from build123d import *

# Parameters (mm, degrees)
SKETCH1_W           = 22
SKETCH1_H           = 37
SKETCH1_R           = 2.5
SKETCH1_W_2         = 12
SKETCH1_H_2         = 10
BOSS_EXTRUDE2_DEPTH = 6
CUT_EXTRUDE2_DEPTH  = 6


with BuildPart() as part:
    # Sketch1 → Boss-Extrude2 (new body)
    with BuildSketch(Plane.XY):
        Rectangle(SKETCH1_W, SKETCH1_H)
        with Locations((-7, 14.5)):
            Circle(SKETCH1_R, mode=Mode.SUBTRACT)
        with Locations((7, 14.5)):
            Circle(SKETCH1_R, mode=Mode.SUBTRACT)
        with Locations((0, -12)):
            Rectangle(SKETCH1_W_2, SKETCH1_H_2, mode=Mode.SUBTRACT)
    extrude(amount=BOSS_EXTRUDE2_DEPTH)

    # Sketch3 → Cut-Extrude2 (cut)
    with BuildSketch(Plane(origin=(0, 0, 0), x_dir=(-1, 0, 0), z_dir=(0, 0, -1))):
        Polygon((0, -17), (-3, -17), (-3, -18.5), (0, -18.5), (3, -18.5), (3, -17), align=None)
    extrude(amount=-CUT_EXTRUDE2_DEPTH, mode=Mode.SUBTRACT)


solid = part.part
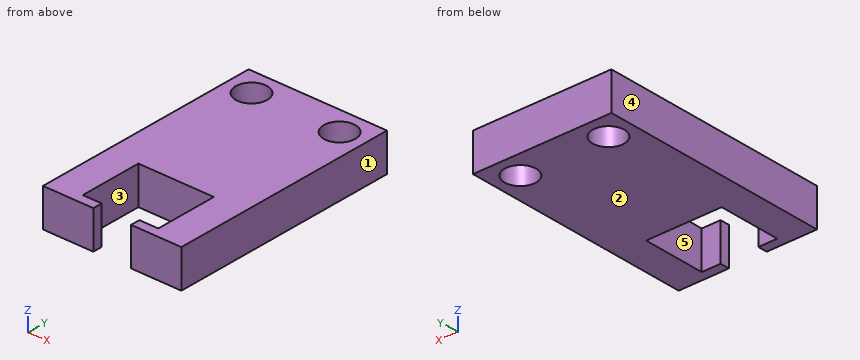
The listing builds one solid part. Answer for the finished solid, in the listing's coordinates (mm). Face numbers are marked on the shaded views. A direction names the side the tool comes from. Give positions to 0.01 mm unless a question says otherwise; leave off trailing zeros. Write each loop counter-clockwise with the first axis right and the second up, starting at its lowest first coordinate (ties: lowest second). Pieces come first, ordered by that corner, then holes. Notation, with made-up numbers: (-36, 8.5) -> (19, 8.5) arc R10 cw to (19, 23.5) -> close; hole circle Ø3 at (32, 43.25). An arc over 180 degrees is marked (long way). One line per question, with ' | ' between items. Start each with the question number.
1. Given pin 1 Ø6 at (x, y) = (-7, 14.5) entering from +Z, flat-ended and moving along its own axis, determine where the tip first touches the part or whether it passes through.
2. Section C-C (z = 1.6) is taken. Determine the outline of the cut face in (x, y), plus the area to 3 significant figures.
3. Section D-D (y = 14.5) is taken. Determine the outline of the cut face in (x, z), plus the area to 3 significant figures.
4. Find the intervals of material crossed by probe 1 along Y at (x, z) = (7, 1.2); probe 2 along X at (y, z) = (15.5, 1.7); probe 3 along X at (y, z) = (14, 4.2), in increasing order.
5. For a pull along X with two mould halves and no side action, classify the marked faces 1, 2 and 3 as pulls with the +X half, pulls with the -X half, needs draft (parallel to the pull), parting line crosses it, or undercut.
6. Section B-B (x = 7) is taken. Determine the outline of the cut face in (y, z), plus the area to 3 significant figures.
7. Section A-A (y = -10) is taken. Determine the outline of the cut face in (x, z).
8. For the marked faces 4 and 5, determine the directions among +Z, -Z, +X, -X, +Y, -Y from which every point of the face is accessible in a straight line to the end or side of a thin tool.
Response values:
1) pin 1: z = 6
2) outline: (-11, -18.5) -> (-3, -18.5) -> (-3, -17) -> (-6, -17) -> (-6, -7) -> (6, -7) -> (6, -17) -> (3, -17) -> (3, -18.5) -> (11, -18.5) -> (11, 18.5) -> (-11, 18.5) -> close; hole circle Ø5 at (-7, 14.5); hole circle Ø5 at (7, 14.5) | area: 646 mm2
3) outline: (-11, 0) -> (-9.5, 0) -> (-9.5, 6) -> (-11, 6) -> close; (-4.5, 0) -> (4.5, 0) -> (4.5, 6) -> (-4.5, 6) -> close; (9.5, 0) -> (11, 0) -> (11, 6) -> (9.5, 6) -> close | area: 72.0 mm2
4) probe 1: -18.5 to 12, 17 to 18.5 | probe 2: -11 to -9.29, -4.71 to 4.71, 9.29 to 11 | probe 3: -11 to -9.45, -4.55 to 4.55, 9.45 to 11
5) face 1: pulls with the +X half | face 2: needs draft | face 3: undercut
6) outline: (-18.5, 0) -> (12, 0) -> (12, 6) -> (-18.5, 6) -> close; (17, 0) -> (18.5, 0) -> (18.5, 6) -> (17, 6) -> close | area: 192 mm2
7) outline: (-11, 0) -> (-6, 0) -> (-6, 6) -> (-11, 6) -> close; (6, 0) -> (11, 0) -> (11, 6) -> (6, 6) -> close
8) face 4: +Z, -Z, -X, +Y, -Y | face 5: +Z, -Z
